from build123d import *
from build123d.topology import SkipClean

# Parameters (mm, degrees)
SKETCH6_R            = 3
SKETCH6_R_2          = 2.19
BOSS_EXTRUDE3_DEPTH  = 2
SKETCH7_W            = 4
SKETCH7_H            = 4
CUT_EXTRUDE2_DEPTH   = 0.5
BOSS_EXTRUDE5_START  = 0.5
BOSS_EXTRUDE5_DEPTH  = 0.5
SKETCH17_R           = 3.5
SKETCH17_R_2         = 3
BOSS_EXTRUDE11_DEPTH = 0.5
BOSS_EXTRUDE12_START = 2
SKETCH18_R           = 3.5
SKETCH18_R_2         = 3.1
BOSS_EXTRUDE12_DEPTH = 2
BOSS_EXTRUDE13_DEPTH = 1.5
SKETCH29_W           = 3
SKETCH29_H           = 3
BOSS_EXTRUDE16_DEPTH = 1.5
SKETCH30_W           = 2.12
SKETCH30_H           = 2.12
CUT_EXTRUDE10_DEPTH  = 2.645512986
SKETCH31_W           = 2.22
SKETCH31_H           = 2.22
BOSS_EXTRUDE17_DEPTH = 1.27
SKETCH32_R           = 0.81
CUT_EXTRUDE11_DEPTH  = 8.729286762
SKETCH33_W           = 3.2
SKETCH33_H           = 3.2
CUT_EXTRUDE12_DEPTH  = 0.18
CIRPATTERN3_COUNT    = 4
SKETCH34_W           = 2.14
SKETCH34_H           = 2.16
CUT_EXTRUDE13_DEPTH  = 2.645512986
SKETCH35_W           = 2.12
SKETCH35_H           = 2.12
CUT_EXTRUDE14_DEPTH  = 2.645512986
SKETCH36_W           = 2.12
SKETCH36_H           = 2.12
CUT_EXTRUDE15_DEPTH  = 2.645512986
CIRPATTERN16_COUNT   = 4
SKETCH37_R           = 10
CUT_EXTRUDE17_DEPTH  = 0.5
SKETCH38_R           = 3.5
SKETCH38_R_2         = 2.85
BOSS_EXTRUDE18_DEPTH = 1.5
SKETCH39_W           = 2.12
SKETCH39_H           = 2.12
CUT_EXTRUDE18_DEPTH  = 0.5
SKETCH40_W           = 8
SKETCH40_H           = 8
SKETCH40_W_2         = 7
SKETCH40_H_2         = 7
BOSS_EXTRUDE19_DEPTH = 2.44
BOSS_EXTRUDE20_START = 0.15
SKETCH41_W           = 8
SKETCH41_H           = 8
SKETCH41_R           = 2.19
BOSS_EXTRUDE20_DEPTH = 0.15
SKETCH42_W           = 8
SKETCH42_H           = 8
SKETCH42_R           = 2.19
BOSS_EXTRUDE21_DEPTH = 0.733937
BOSS_EXTRUDE21_DRAFT = 45
SKETCH43_W           = 7.12
SKETCH43_H           = 7.12
CUT_EXTRUDE19_DEPTH  = 10


with BuildPart() as part:
    # Sketch6 → Boss-Extrude3 (new body)
    with BuildSketch(Plane(origin=(0, 0, 0), x_dir=(1, 0, 0), z_dir=(0, 1, 0))):
        with Locations(Location((0, 0, 0), (0, 0, 270))):
            Circle(SKETCH6_R)
        with Locations(Location((0, 0, 0), (0, 0, 270))):
            Circle(SKETCH6_R_2, mode=Mode.SUBTRACT)
    extrude(amount=BOSS_EXTRUDE3_DEPTH)

    # Sketch7 → Cut-Extrude2 (cut)
    with BuildSketch(Plane(origin=(0, 0, 0), x_dir=(-1, 0, 0), z_dir=(0, -1, 0))):
        Rectangle(SKETCH7_W, SKETCH7_H)
    extrude(amount=-CUT_EXTRUDE2_DEPTH, mode=Mode.SUBTRACT)

    # Sketch8 → Boss-Extrude5 (add)
    with BuildSketch(Plane(origin=(0, 0.5, 0), x_dir=(-1, 0, 0), z_dir=(0, -1, 0)).offset(BOSS_EXTRUDE5_START)):
        with BuildLine():
            Line((-0.892244361, 2), (0.892244361, 2))
            ThreePointArc((0.892244361, 2), (0, 2.19), (-0.892244361, 2))
        make_face()
        with BuildLine():
            Line((-2, 0.892244361), (-2, -0.892244361))
            ThreePointArc((-2, -0.892244361), (-2.19, 0), (-2, 0.892244361))
        make_face()
        with BuildLine():
            Line((-0.892244361, -2), (0.892244361, -2))
            ThreePointArc((0.892244361, -2), (0, -2.19), (-0.892244361, -2))
        make_face()
        with BuildLine():
            Line((2, 0.892244361), (2, -0.892244361))
            ThreePointArc((2, -0.892244361), (2.19, 0), (2, 0.892244361))
        make_face()
    extrude(amount=-BOSS_EXTRUDE5_DEPTH)

    # Sketch17 → Boss-Extrude11 (add)
    with BuildSketch(Plane(origin=(0, 0, 0), x_dir=(-1, 0, 0), z_dir=(0, -1, 0))):
        with Locations(Location((0, 0, 0), (0, 0, 90))):
            Circle(SKETCH17_R)
        with Locations(Location((0, 0, 0), (0, 0, 90))):
            Circle(SKETCH17_R_2, mode=Mode.SUBTRACT)
    extrude(amount=-BOSS_EXTRUDE11_DEPTH)

    # Sketch18 → Boss-Extrude12 (add)
    with BuildSketch(Plane(origin=(0, 0, 0), x_dir=(-1, 0, 0), z_dir=(0, -1, 0)).offset(BOSS_EXTRUDE12_START)):
        with Locations(Location((0, 0, 0), (0, 0, 90))):
            Circle(SKETCH18_R)
        with Locations(Location((0, 0, 0), (0, 0, 90))):
            Circle(SKETCH18_R_2, mode=Mode.SUBTRACT)
    extrude(amount=-BOSS_EXTRUDE12_DEPTH)

    # Sketch19 → Boss-Extrude13 (add, symmetric)
    with BuildSketch(Plane.XY):
        Polygon((4.288855584, -2), (5.121320344, -1.167535241), (3, 0.953785103), (2.19, 0.143785103), (3.250660172, -0.916875069), (3.250660172, -2), (4.033756176, -2), align=None)
    boss_extrude13 = extrude(amount=BOSS_EXTRUDE13_DEPTH, both=True)

    # Sketch29 → Boss-Extrude16 (add)
    with BuildSketch(Plane(origin=(1.976892551, 1.976892551, 0), x_dir=(0, 0, -1), z_dir=(0.707106781186548, 0.7071067811865471, 0))):
        with Locations((0, -2.94689243)):
            Rectangle(SKETCH29_W, SKETCH29_H)
    boss_extrude16 = extrude(amount=BOSS_EXTRUDE16_DEPTH)

    # Sketch30 → Cut-Extrude10 (cut)
    with BuildSketch(Plane(origin=(3.037552723, 3.037552723, 0), x_dir=(0, 0, -1), z_dir=(0.707106781186548, 0.7071067811865471, 0))):
        with Locations((0, -2.94689243)):
            Rectangle(SKETCH30_W, SKETCH30_H)
    extrude(amount=-CUT_EXTRUDE10_DEPTH, mode=Mode.SUBTRACT)

    # Sketch31 → Boss-Extrude17 (add)
    with BuildSketch(Plane(origin=(1.166892551, 1.166892551, 0), x_dir=(0, 0, 1), z_dir=(-0.7071067811865441, -0.7071067811865509, 0))):
        with Locations((-0.05, -2.89689243)):
            Rectangle(SKETCH31_W, SKETCH31_H)
    boss_extrude17 = extrude(amount=-BOSS_EXTRUDE17_DEPTH)

    # Sketch32 → Cut-Extrude11 (cut, symmetric)
    with BuildSketch(Plane(origin=(2.064918163, 2.064918163, 0), x_dir=(0, 0, -1), z_dir=(0.7071067811865444, 0.7071067811865508, 0))):
        with Locations(Location((0, -2.94689243, 0), (0, 0, 155.306163656))):
            Circle(SKETCH32_R)
    cut_extrude11 = extrude(amount=CUT_EXTRUDE11_DEPTH, both=True, mode=Mode.SUBTRACT)

    # Sketch33 → Cut-Extrude12 (cut)
    with BuildSketch(Plane(origin=(3.037552723, 3.037552723, 0), x_dir=(0, 0, -1), z_dir=(0.707106781186548, 0.7071067811865471, 0))):
        with Locations((0, -2.94689243)):
            Rectangle(SKETCH33_W, SKETCH33_H)
    cut_extrude12 = extrude(amount=-CUT_EXTRUDE12_DEPTH, mode=Mode.SUBTRACT)

    # CirPattern3: Boss-Extrude13, Boss-Extrude16 ×4 about axis
    cirpattern3_axis = Axis((0, 0, 0), (0, 1, 0))
    add([boss_extrude13.rotate(cirpattern3_axis, i * 360 / CIRPATTERN3_COUNT) for i in range(1, CIRPATTERN3_COUNT)])
    add([boss_extrude16.rotate(cirpattern3_axis, i * 360 / CIRPATTERN3_COUNT) for i in range(1, CIRPATTERN3_COUNT)])

    # Sketch34 → Cut-Extrude13 (cut)
    with BuildSketch(Plane(origin=(-3.037552723, 3.037552723, 0), x_dir=(0, 0, 1), z_dir=(-0.707106781186548, 0.7071067811865471, 0))):
        with Locations((0, -2.94689243)):
            Rectangle(SKETCH34_W, SKETCH34_H)
    extrude(amount=-CUT_EXTRUDE13_DEPTH, mode=Mode.SUBTRACT)

    # Sketch35 → Cut-Extrude14 (cut)
    with BuildSketch(Plane(origin=(0, 3.037552723, -3.037552723), x_dir=(1, 0, 0), z_dir=(7.355440612690688e-15, 0.7071067811865471, -0.707106781186548))):
        with Locations((0, 2.94689243)):
            Rectangle(SKETCH35_W, SKETCH35_H)
    extrude(amount=-CUT_EXTRUDE14_DEPTH, mode=Mode.SUBTRACT)

    # Sketch36 → Cut-Extrude15 (cut)
    with BuildSketch(Plane(origin=(0, 3.037552723, 3.037552723), x_dir=(1, 0, 0), z_dir=(-2.417740350526155e-15, 0.7071067811865471, 0.707106781186548))):
        with Locations((0, -2.94689243)):
            Rectangle(SKETCH36_W, SKETCH36_H)
    extrude(amount=-CUT_EXTRUDE15_DEPTH, mode=Mode.SUBTRACT)

    # CirPattern16: Boss-Extrude17, Cut-Extrude11, Cut-Extrude12 ×4 about axis
    cirpattern16_axis = Axis((0, 0, 0), (0, 1, 0))
    add([boss_extrude17.rotate(cirpattern16_axis, i * 360 / CIRPATTERN16_COUNT) for i in range(1, CIRPATTERN16_COUNT)])
    add([cut_extrude11.rotate(cirpattern16_axis, i * 360 / CIRPATTERN16_COUNT) for i in range(1, CIRPATTERN16_COUNT)], mode=Mode.SUBTRACT)
    add([cut_extrude12.rotate(cirpattern16_axis, i * 360 / CIRPATTERN16_COUNT) for i in range(1, CIRPATTERN16_COUNT)], mode=Mode.SUBTRACT)

    # Sketch37 → Cut-Extrude17 (cut)
    with BuildSketch(Plane.XZ.offset(2)):
        Circle(SKETCH37_R)
    extrude(amount=-CUT_EXTRUDE17_DEPTH, mode=Mode.SUBTRACT)

    # Sketch38 → Boss-Extrude18 (add)
    with SkipClean():  # the faces are left unmerged after this step: merging them gives an invalid solid
        with BuildSketch(Plane(origin=(0, 0.5, 0), x_dir=(1, 0, 0), z_dir=(0, 1, 0))):
            with Locations(Location((0, 0, 0), (0, 0, 111.75765302))):
                Circle(SKETCH38_R)
            Circle(SKETCH38_R_2, mode=Mode.SUBTRACT)
        extrude(amount=BOSS_EXTRUDE18_DEPTH)
    add(part.part.scale(1), mode=Mode.REPLACE)  # the faces are merged on a copy

    # Sketch39 → Cut-Extrude18 (cut)
    with BuildSketch(Plane(origin=(0, 2.064918163, -2.064918163), x_dir=(1, 0, 0), z_dir=(-2.4688501310822543e-15, 0.7071067811865508, -0.7071067811865444))):
        with Locations((0, 2.94689243)):
            Rectangle(SKETCH39_W, SKETCH39_H)
    extrude(amount=CUT_EXTRUDE18_DEPTH, mode=Mode.SUBTRACT)



with BuildPart() as body_2:
    # Sketch40 → Boss-Extrude19 (new body)
    with BuildSketch(Plane(origin=(0, 2, 0), x_dir=(1, 0, 0), z_dir=(0, 1, 0))):
        Rectangle(SKETCH40_W, SKETCH40_H)
        Rectangle(SKETCH40_W_2, SKETCH40_H_2, mode=Mode.SUBTRACT)
    extrude(amount=BOSS_EXTRUDE19_DEPTH)


with BuildPart() as part_1:
    with SkipClean():  # the faces are left unmerged after this step: merging them gives an invalid solid
        add(part.part)

        add(body_2.part)  # Boss-Extrude20 merges body 2
        # Sketch41 → Boss-Extrude20 (add)
        with BuildSketch(Plane.XZ.offset(-2).offset(BOSS_EXTRUDE20_START)):
            Rectangle(SKETCH41_W, SKETCH41_H)
            with Locations(Location((0, 0, 0), (0, 0, 294.042710138))):
                Circle(SKETCH41_R, mode=Mode.SUBTRACT)
        extrude(amount=-BOSS_EXTRUDE20_DEPTH)


with BuildPart() as boss_extrude21_tool:
    # Sketch42 → Boss-Extrude21 (with draft: the straight prism first)
    with BuildSketch(Plane.XZ.offset(-1.85)):
        Rectangle(SKETCH42_W, SKETCH42_H)
        with Locations(Location((0, 0, 0), (0, 0, 294.042710138))):
            Circle(SKETCH42_R, mode=Mode.SUBTRACT)
    extrude(amount=BOSS_EXTRUDE21_DEPTH)
    # Boss-Extrude21: the draft: its side faces are tilted about the plane it starts from
    boss_extrude21_sides = [boss_extrude21_tool.faces().sort_by_distance(p)[0] for p in [
        (-4, 1.4830315, 0),
        (0, 1.4830315, -4),
        (4, 1.4830315, 0),
        (0, 1.4830315, 4),
        (-0.892244361, 1.4830315, 2),
    ]]
    draft(boss_extrude21_sides, Plane.XZ.offset(-1.85), BOSS_EXTRUDE21_DRAFT)


with BuildPart() as part_2:
    add(part_1.part)

    # Boss-Extrude21: add boss_extrude21_tool
    add(boss_extrude21_tool.part)

    # Sketch43 → Cut-Extrude19 (cut)
    with BuildSketch(Plane(origin=(0, 2, 0), x_dir=(1, 0, 0), z_dir=(0, 1, 0))):
        Rectangle(SKETCH43_W, SKETCH43_H)
    extrude(amount=CUT_EXTRUDE19_DEPTH, mode=Mode.SUBTRACT)


solid = part_2.part
Part model, mm, in its own coordinate system. A direction names the side the tool comes from. Coordinates: 2 decimals unless noted, no trailing zeros. Loops run counter-clockwise (first coordinate to the right, second up) from the corner with the lowest first, then second, coordinate; pieces in that order, holes last. Notation, with made-up numbers: (7.25, 9.25) - (22.25, 9.25) arc R20 ccw to (22.25, 16.25) - close; hole circle Ø8 at (77.25, -34.5). An arc over 180 degrees is marked (long way). Write each question's results on one line, items separated by ' | '. Start each with the question number.
Q1. Which spindle directions (+Z, -Z, +X, -X, +Y, -Y) get a long thin tool onto all of the face, cutting with end or side? Do faces 4 (the flat face through (-1.7, 0.5, -1.7)), 5 (the flat face through (3, 1.116, 3)), 6 (the flat face through (-0.015, -0.34, 5.327)), 7 (the flat face through (-3, 1.116, 3)). Say none if no direction does.
Q2. Probe line 1 along Z through (x, y) = (-5, 0.3); line 2 along X through (y, z) = (1.9, 0); line 3 along X through (y, z) = (3.75, 1.5). List the from-to ranges inside material, lowest first.
Q3. Two-plate mould, pull along X, no slides. Class faces 1 (the flat face through (1.5, 0, 4)), 2 (the cylindrical face through (2.175, -0.927, -2.209)), 3 (the flat face through (-0.021, -0.105, 5.925)): +X half, -X half, draft (parallel to the pull), parting line (faces both ways), or undercut.
Q4. Slice it at B-B on z = -2.5. Give the cut face in (x, y), and give its area (3 significant figures).
Q5. Slice it at D-D on z = -5.5. Give the cut face in (x, y), and give its area (3 significant figures).
Q6. Drop flat-ended pins along their axis: pin 1 Ø0.6 at (y, z) = (0, -4.5) entering from -X; pin 2 Ø0.7 at (y, z) = (3, -0.5) entering from -X; pin 3 Ø1 at (y, z) = (0.5, 1) entering from +X. Give the stop position or say it passes through.
Q7. Slice it at C-C on x = -0.5. Give the number of separate pieces and of enclosed holes in the cut face, and give its area (3 significant figures).
Q8. Slice it at A-A on y = 3. Give the cut face in (x, z).
Answer:
1) face 4: -Y | face 5: +Z, +X, -Y | face 6: +Y | face 7: +Z, -X, -Y
2) line 1: z = -1.5 to -1.07, 1.07 to 1.5 | line 2: x = -4 to -2.19, 2.19 to 4 | line 3: x = -4 to -3.56, 3.56 to 4
3) face 1: +X half | face 2: undercut | face 3: draft
4) outline: (-4, 1.85) - (-3.27, 1.12) - (-2.45, 1.12) - (-2.45, -1.5) - (-1.83, -1.5) - (-1.83, 0) - (-1.5, 0) - (-1.5, -0.17) - (1.5, -0.17) - (1.5, 0) - (1.83, 0) - (1.83, -1.5) - (2.45, -1.5) - (2.45, 1.12) - (3.27, 1.12) - (4, 1.85) - (4, 4.44) - (3.56, 4.44) - (3.56, 2) - (-3.56, 2) - (-3.56, 4.44) - (-4, 4.44) - close | area: 16.5 mm2
5) outline: (-1.5, -0.79) - (1.5, -0.79) - (1.5, 0.32) - (1.06, 0.32) - (1.06, -0.17) - (-1.06, -0.17) - (-1.06, 0.32) - (-1.5, 0.32) - close | area: 2.30 mm2
6) pin 1: stops at x = -1.5 | pin 2: stops at x = -4 | pin 3: stops at x = 5.82
7) separate pieces: 4 | enclosed holes: 0 | area: 12.1 mm2
8) outline: (-4, -4) - (4, -4) - (4, 4) - (-4, 4) - close; hole (-3.56, -3.56) - (3.56, -3.56) - (3.56, 3.56) - (-3.56, 3.56) - close
